Autodesk Inventor part; units mm, degrees
ref_plane "YZ Plane" through (0, 0, 0) normal (1, 0, 0) x (0, 1, 0)
ref_plane "XZ Plane" through (0, 0, 0) normal (0, 1, 0) x (-1, 0, 0)
ref_plane "XY Plane" through (0, 0, 0) normal (0, 0, 1) x (1, 0, 0)
sketch "Sketch1" plane through (0, 0, 0) normal (0, 0, 1) x (1, 0, 0)
  circle A0 centre (0, 0) radius 25.4
  circle A1 centre (0, 0) radius 9.5631
  dimension "d0" = 50.8
  dimension "d4" = 19.1262
extrude "Extrusion1" add sketch "Sketch1" along normal blind 6.35
sketch "Sketch2" plane through (0, 0, 6.35) normal (0, 0, 1) x (1, 0, 0)
  circle A0 centre (0, 0) radius 17.5641 construction
  line L0 (0, 17.5641) -> (0, 0) construction
  line L1 (0, 0) -> (-8.782, 15.211) construction
  line L2 (0, 0) -> (0, -17.5641) construction
  line L3 (0, 0) -> (8.7821, -15.211) construction
  circle A1 centre (0, 0) radius 12.7 construction
  arc A2 (0, 12.7) -> (-6.35, 10.9985) centre (0, 0) ccw
  arc A3 (0, 17.5641) -> (-8.782, 15.211) centre (0, 0) ccw
  line L4 (-8.782, 15.211) -> (-6.35, 10.9985)
  line L5 (0, 12.7) -> (0, 17.5641)
  dimension "d5" = 35.1282
  dimension "d6" = 30
  dimension "d7" = 25.4
extrude "Extrusion3" cut sketch "Sketch2" against normal up to surface (6.35 mm away)
pattern_circular "Circular Pattern2" count 4 over 360 about axis through (0, 0, 0) along (0, 0, 1) of "Extrusion3"
fillet "Fillet1" radius 1.27 8 edges at (0, 17.5641, 3.175) (0, 12.7, 3.175) (17.5641, 0, 3.175) (12.7, 0, 3.175) (0, -17.5641, 3.175) (0, -12.7, 3.175) (-17.5641, 0, 3.175) (-12.7, 0, 3.175)
fillet "Fillet2" radius 2.54 2 edges at (-25.4, 0, 0) (-25.4, 0, 6.35)
properties part number "Spool Cap Section Mk1"
For this review, take the finished solid that the model builds, in its own axes (mm). Round coordinates to 2 decimals unless told otherwise and drop trailing zeros. Loops run counter-clockwise (first coordinate to the right, second up) from the corner with the lowest first, then second, coordinate; pieces in that order, holes last.
(1) Clearance check with flat-ended pins moving along their axes: P1, Ø1.2, axis at y = 15.5, z = 2.5, coming from the -X side; P2, Ø1.5, axis at y = -7.5, z = 2, coming from the +X side; P3, Ø1.9, axis at x = 15.5, z = 2, coming from the +Y side. State where each tip first meets the part, or that it passes through.
Returned:
P1: stops at x = -20.57
P2: stops at x = 24.46
P3: stops at y = 20.78
(2) We need section B-B (x = -2). State how many separate pieces and enclosed holes the cut face has, plus the area to 3 significant figures.
Returned:
separate pieces: 3
enclosed holes: 0
area: 166 mm2
(3) We need section C-C (z = 1.5). Give the boundary of the cut face in (x, y), plus the area to 3 significant figures.
Returned:
outline: circle Ø50.35 at (0, 0); hole (-17.51, -1.37) arc R17.56 ccw to (-15.21, -8.78) - (-11, -6.35) arc R12.7 cw to (-12.65, -1.15) arc R1.27 ccw to (-13.91, 0) - (-16.24, 0) arc R1.27 ccw to start; hole circle Ø19.13 at (0, 0); hole (-8.78, 15.21) - (-6.35, 11) arc R12.7 cw to (-1.15, 12.65) arc R1.27 ccw to (0, 13.91) - (0, 16.24) arc R1.27 ccw to (-1.37, 17.51) arc R17.56 ccw to start; hole (0, -16.24) arc R1.27 ccw to (1.37, -17.51) arc R17.56 ccw to (8.78, -15.21) - (6.35, -11) arc R12.7 cw to (1.15, -12.65) arc R1.27 ccw to (0, -13.91) - close; hole (11, 6.35) arc R12.7 cw to (12.65, 1.15) arc R1.27 ccw to (13.91, 0) - (16.24, 0) arc R1.27 ccw to (17.51, 1.37) arc R17.56 ccw to (15.21, 8.78) - close
area: 1,550 mm2
(4) Wall thickness on line 1 along Y through (x, z) = (7.5, 5.25); line 2 along X through (y, z) = (-6, 6); line 3 along X through (y, z) = (-6.5, 4.5): over which ranges is each line inside the solid? List them lowest first.
Returned:
line 1: y = -23.8 to -15.88, -12.99 to -5.93, 5.93 to 23.8
line 2: x = -23.39 to -16.51, -11.19 to -7.45, 7.45 to 23.39
line 3: x = -24.46 to -16.32, -11.26 to -7.01, 7.01 to 24.46
(5) We need section A-A (z = 5.5). Give the boundary of the cut face in (x, y), plus the area to 3 significant figures.
Returned:
outline: circle Ø49.51 at (0, 0); hole (-17.51, -1.37) arc R17.56 ccw to (-15.21, -8.78) - (-11, -6.35) arc R12.7 cw to (-12.65, -1.15) arc R1.27 ccw to (-13.91, 0) - (-16.24, 0) arc R1.27 ccw to start; hole circle Ø19.13 at (0, 0); hole (-8.78, 15.21) - (-6.35, 11) arc R12.7 cw to (-1.15, 12.65) arc R1.27 ccw to (0, 13.91) - (0, 16.24) arc R1.27 ccw to (-1.37, 17.51) arc R17.56 ccw to start; hole (0, -16.24) arc R1.27 ccw to (1.37, -17.51) arc R17.56 ccw to (8.78, -15.21) - (6.35, -11) arc R12.7 cw to (1.15, -12.65) arc R1.27 ccw to (0, -13.91) - close; hole (11, 6.35) arc R12.7 cw to (12.65, 1.15) arc R1.27 ccw to (13.91, 0) - (16.24, 0) arc R1.27 ccw to (17.51, 1.37) arc R17.56 ccw to (15.21, 8.78) - close
area: 1,490 mm2
(6) Mouldability with a two-part tool opening along X and no side actions: class faces 1 (the cylindrical face through (-12.117, -3.805, 3.219)), 2 (the flat face through (0, -10, 0)), 3 (the flat face through (-15, 0, 3)) as released by +X, released by -X, zero draft, split by the parting line, or undercut.
Returned:
face 1: undercut
face 2: zero draft
face 3: undercut
